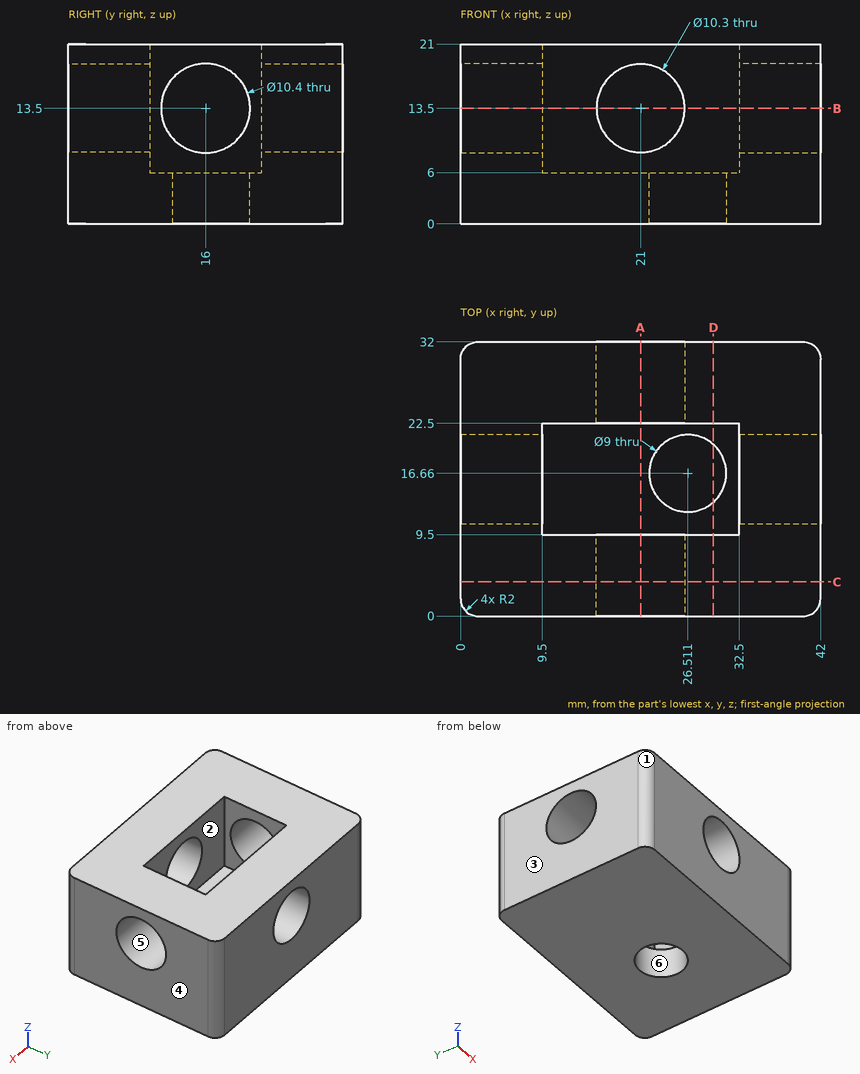
Study the drawing (mm; zero at the part's minimum x, y, z) and answer. A direction names the side the tool comes from. Coordinates: 2 decimals unless noted, no trailing zeros. Order: outer loops, then holes, each group sorted by start corner. A loop starts at its lowest first (then second) coordinate and runs counter-clockwise, first axis right, second up. Notation, with made-up numbers: M -18.75,-21.5 L -4.75,-21.5 A25 cw -4.75,9.5 Z; hole C -21.75,-22.75 d9. An arc over 180 degrees is marked long. Answer as a JSON object with one key per item and string values. Group by question number.
1. Determine the mould class of the marked faces 3, 4, 5 and 6 for opening direction X: released by +X, released by -X, zero draft, split by the parting line, or undercut.
2. Section A-A on x = 21 is taken. Write down the section's boundary in (y, z).
3. A tool of negligible diameter and unlimited length cuts with its end or side. For the marked faces 1 and 2, from which of +Z, -Z, +X, -X, +Y, -Y can it reach the whole face along a straight path? Write none if from no direction.
4. Section D-D on x = 29.5 is taken. Write down the section's boundary in (y, z) (1 decimal), then the cut area to 3 significant figures.
5. Section C-C on y = 4 is taken. Write down the section's boundary in (x, z).
6. Straight lines are drawn through the part: line 1 (Y direction, x = 26, z = 16); line 2 (Z direction, x = 35.5, y = 16); line 3 (Z direction, x = 21, y = 4). For each, find the intervals that lie inside material, in ascending order.
7. Section B-B on z = 13.5 is taken. Write down the section's boundary in (x, y).
8. Flat-ended cylindrical pins translate along their axes: P1, Ø4, axis at x = 16.5, y = 17.5, coming from the +Z side; P2, Ø12, axis at y = 16, z = 13.5, coming from the +X side; P3, Ø8, axis at x = 26.51, y = 16.66, coming from the +Z side (3 decimals). Find the tip coordinate at first contact, or state that the pin passes through.
Values follow:
{
 "1": {"face 3": "released by -X", "face 4": "released by +X", "face 5": "zero draft", "face 6": "undercut"},
 "2": {"outline": "M 0,0 L 32,0 L 32,8.35 L 22.5,8.35 L 22.5,6 L 9.5,6 L 9.5,8.35 L 0,8.35 Z; M 0,18.65 L 9.5,18.65 L 9.5,21 L 0,21 Z; M 22.5,18.65 L 32,18.65 L 32,21 L 22.5,21 Z"},
 "3": {"face 1": "+Z, -Z, -X, -Y", "face 2": "+Z"},
 "4": {"outline": "M 0,0 L 13.3,0 L 13.3,6 L 9.5,6 L 9.5,21 L 0,21 Z; M 20,0 L 32,0 L 32,21 L 22.5,21 L 22.5,6 L 20,6 Z", "area": "437 mm2"},
 "5": {"outline": "M 0,0 L 42,0 L 42,21 L 0,21 Z; hole C 21,13.5 d10.3"},
 "6": {"line 1": "0 to 9.5, 22.5 to 32", "line 2": "0 to 8.3, 18.7 to 21", "line 3": "0 to 8.35, 18.65 to 21"},
 "7": {"outline": "M 0,2 A2 ccw 2,0 L 15.85,0 L 15.85,9.5 L 9.5,9.5 L 9.5,10.8 L 0,10.8 Z; M 0,21.2 L 9.5,21.2 L 9.5,22.5 L 15.85,22.5 L 15.85,32 L 2,32 A2 ccw 0,30 Z; M 26.15,0 L 40,0 A2 ccw 42,2 L 42,10.8 L 32.5,10.8 L 32.5,9.5 L 26.15,9.5 Z; M 26.15,22.5 L 32.5,22.5 L 32.5,21.2 L 42,21.2 L 42,30 A2 ccw 40,32 L 26.15,32 Z"},
 "8": {"P1": "z = 6", "P2": "x = 42", "P3": "through"}
}
